Design review of the part built by this model. Coordinates are the model's own, in mm. Coordinates: 2 decimals unless noted, no trailing zeros. Write each loop counter-clockwise with the first axis right and the second up, starting at its lowest first coordinate (ties: lowest second). Pieces come first, ordered by that corner, then holes.
Q1. Take a section at A-A (x = 0). State how many separate pieces and enclosed holes the cut face has, and give its area (3 significant figures).
Q2. Take a section at B-B (z = -5). Give the boundary of the cut face in (x, y).
Q3. For probe 1 along Z at (x, y) = (-0.25, -0.5); probe 2 along Z at (x, y) = (-1, -0.5); probe 3 along Y at (x, z) = (-0.25, -7), list the stretches that pass through material, from the lowest coordinate up.
Q4. Insertion check: pin 1 (2 mm diameter, centred on y = -1.5, z = 19.5, fed in from -X); pin 2 (2 mm diameter, centred on x = 1.5, z = -16, fed in from +Y); pin 3 (2 mm diameter, centred on x = -1.5, y = -3, fed in from +Z). Each pin has a flat end and moves straight along its axis. Give the tip position at first contact, or say it passes through.
Autodesk Inventor part; units mm, degrees
ref_plane "YZ Plane" through (0, 0, 0) normal (1, 0, 0) x (0, 1, 0)
ref_plane "XZ Plane" through (0, 0, 0) normal (0, 1, 0) x (-1, 0, 0)
ref_plane "XY Plane" through (0, 0, 0) normal (0, 0, 1) x (1, 0, 0)
sketch "Sketch1" plane through (0, 0, 0) normal (0, 0, 1) x (1, 0, 0)
  circle A0 centre (0, 0) radius 3.6
  dimension "d0" = 7.2
extrude "Extrusion1" add sketch "Sketch1" along normal mid plane 83.2
sketch "Sketch2" plane through (0, 0, -41.6) normal (0, 0, -1) x (-1, 0, 0)
  circle A0 centre (0, 0) radius 3.6
  circle A1 centre (0, 0) radius 3.6
  line L0 (3.1168, -1.8015) -> (-3.1186, -1.7985)
  dimension "d3" = 1.8
extrude "Extrusion2" cut sketch "Sketch2" against normal blind 14.4 contours L0 A0 picked at (0.0258, -2.6154)
sketch "Sketch3" plane through (3.1186, -1.7985, -41.6) normal (0.0005, -1, 0) x (1, 0.0005, 0)
  line L0 (-3.1177, -16.64) -> (-3.1177, 99.84)
  circle A0 centre (-3.1177, 3.2) radius 1.2
  line L1 (0, 0) -> (-6.2354, 0)
  point P0 (-3.1177, 41.6)
  dimension "d6" = 2.4
  dimension "d7" = 3.2
extrude "Extrusion3" cut sketch "Sketch3" against normal blind 14.4
mirror "Mirror1" about plane through (0, 0, 0) normal (0, 0, 1) of "Extrusion3", "Extrusion2"
sketch "Sketch4" plane through (0, 0, 0) normal (1, 0, 0) x (0, 1, 0)
  line L0 (-3.6, -27.2) -> (-3.6, 27.2)
  line L1 (-1.7985, -27.2) -> (-3.6, -27.2)
  line L2 (-1.7985, -27.2) -> (-3.6, -25.3985)
  point P0 (0, 0)
  point P1 (-1.8015, -27.2)
  dimension "d10" = 45
extrude "Extrusion4" cut sketch "Sketch4" along normal mid plane 14.4
sketch "Sketch5" plane through (0, 0, -41.6) normal (0, 0, -1) x (-1, 0, 0)
  point P0 (0, 0)
sketch "Sketch6" plane through (0, 0, -41.6) normal (0, 0, -1) x (-1, 0, 0)
  line L0 (-3.1186, -1.7985) -> (3.1168, -1.8015)
  arc A0 (3.1168, -1.8015) -> (-3.1186, -1.7985) centre (0, 0) ccw
  line L1 (-3.1186, -1.7985) -> (3.1168, -1.8015)
  arc A1 (3.1168, -1.8015) -> (-3.1186, -1.7985) centre (0, 0) ccw
  line L2 (5.2617, -6.8026) -> (-5.2683, -6.7974)
  arc A2 (5.2617, -6.8026) -> (-5.2683, -6.7974) centre (0, 0) ccw
  dimension "d13" = 5
extrude "Extrusion5" [suppressed]
properties part number "Back axle"
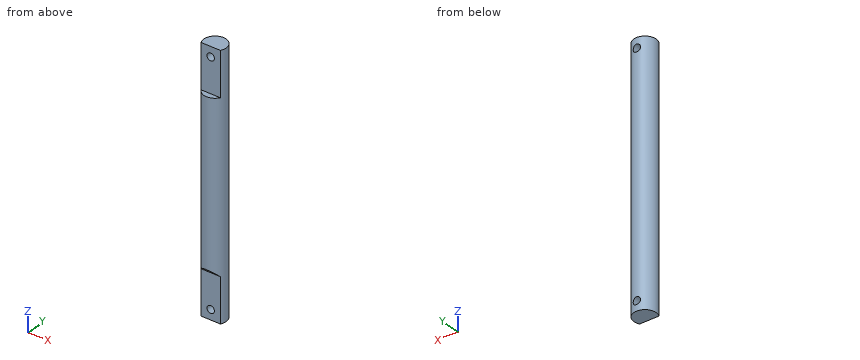
Response:
1. separate pieces: 3
1. enclosed holes: 0
1. area: 520 mm2
2. outline: circle Ø7.2 at (0, 0)
3. probe 1: z = -41.6 to -39.57, -37.23 to 37.23, 39.57 to 41.6
3. probe 2: z = -41.6 to -39.06, -37.74 to 37.74, 39.06 to 41.6
3. probe 3: y = -3.59 to 3.59
4. pin 1: stops at x = -3.57
4. pin 2: stops at y = 3.57
4. pin 3: stops at z = 27.2
